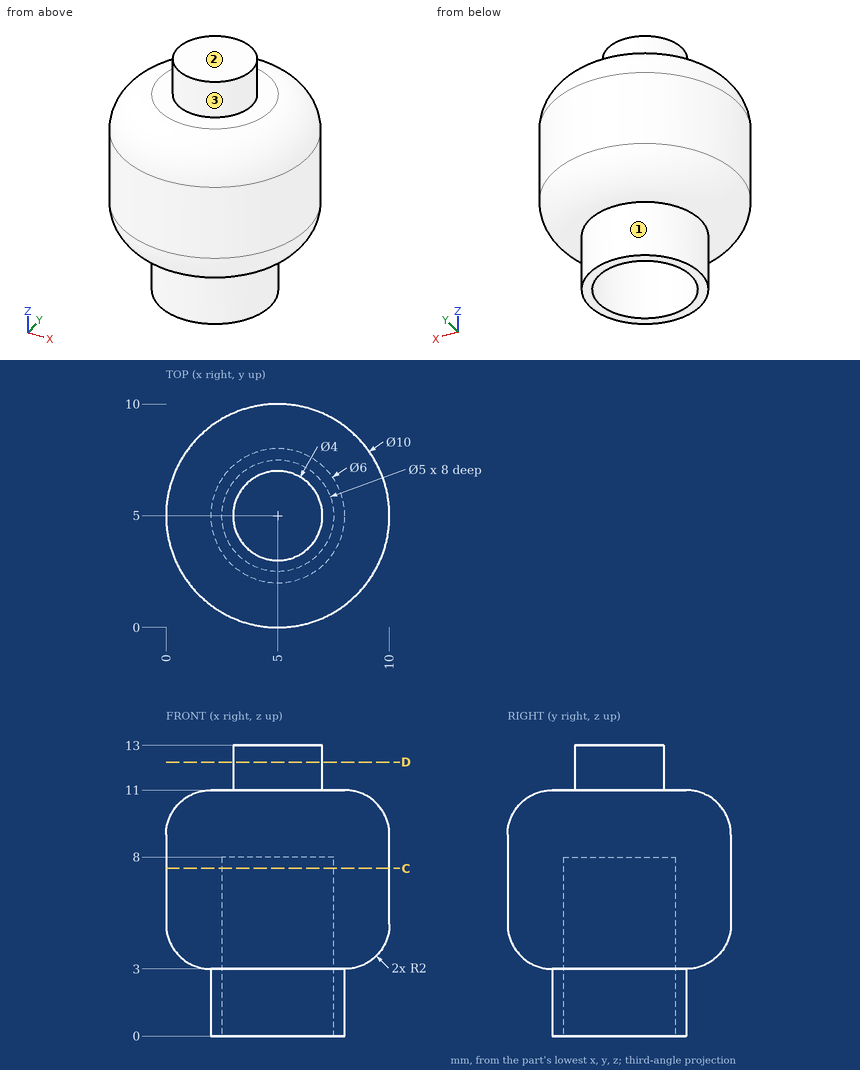
Could you check a few things on this drawing? It's one solid part, dimensions in mm from its lowest x, y, z. A direction names the side the tool comes from. Round coordinates to 2 decimals unless told otherwise and drop trailing zeros. Loops run counter-clockwise (first coordinate to the right, second up) from the corner with the lowest first, then second, coordinate; pieces in that order, holes last. Notation, with made-up numbers: (46, -15) -> (67, -15) arc R26 cw to (67, 0) -> close; hole circle Ø1 at (80, 83). An arc over 180 degrees is marked (long way). One line per item, written item: value. Start each with the question number.
1. For the marked faces 1, 2 and 3, which set-ups out of +Z, -Z, +X, -X, +Y, -Y let a thin tool reach every point of the face, with its end or its side?
2. If we section it at D-D, the plane z = 12.25: Write out the boundary of the cut face in (x, y), then the cut area to 3 significant figures.
3. If I drill on probe 1 along Y at (x, z) = (5, 5.25); probe 2 along X at (y, z) = (4, 7); probe 3 along Y at (x, z) = (3.5, 6.75), over which ranges is the centre line in solid material (lowest first)?
4. For pin 1 (6 mm diameter, centred on x = 7.5, z = 11.5, fed in from -Y); pin 2 (4 mm diameter, centred on x = 7.5, y = 1.5, fed in from +Z); pin 3 (1.5 mm diameter, centred on x = 5.5, y = 4.5, fed in from -Z), each with a flat end and sliding along its axis, tell me the tip position at first contact or that it passes through.
5. If we section it at C-C, the plane z = 7.5: Write out the boundary of the cut face in (x, y).
Calculated:
1. face 1: -Z
1. face 2: +Z, +X, -X, +Y, -Y
1. face 3: +Z
2. outline: circle Ø4 at (5, 5)
2. area: 12.6 mm²
3. probe 1: y = 0 to 2.5, 7.5 to 10
3. probe 2: x = 0.1 to 2.71, 7.29 to 9.9
3. probe 3: y = 0.23 to 3, 7 to 9.77
4. pin 1: stops at y = 0.04
4. pin 2: stops at z = 11
4. pin 3: stops at z = 8
5. outline: circle Ø10 at (5, 5); hole circle Ø5 at (5, 5)
